The drawing under review shows one solid part. Ordinate dimensions are in mm from its lowest x, y, z. A direction names the side the tool comes from. Coordinates: 2 decimals unless noted, no trailing zeros. Order: outer loops, then holes, each group sorted by start corner. A loop starts at its lowest first (then second) coordinate and runs counter-clockwise, first axis right, second up. Notation, with made-up numbers: (-29, -12.5) - (16, -12.5) arc R31 cw to (16, 23.5) - close; hole circle Ø7 at (46.5, 84). An arc over 180 degrees is marked (long way). Answer in a Markdown table with one row per item.
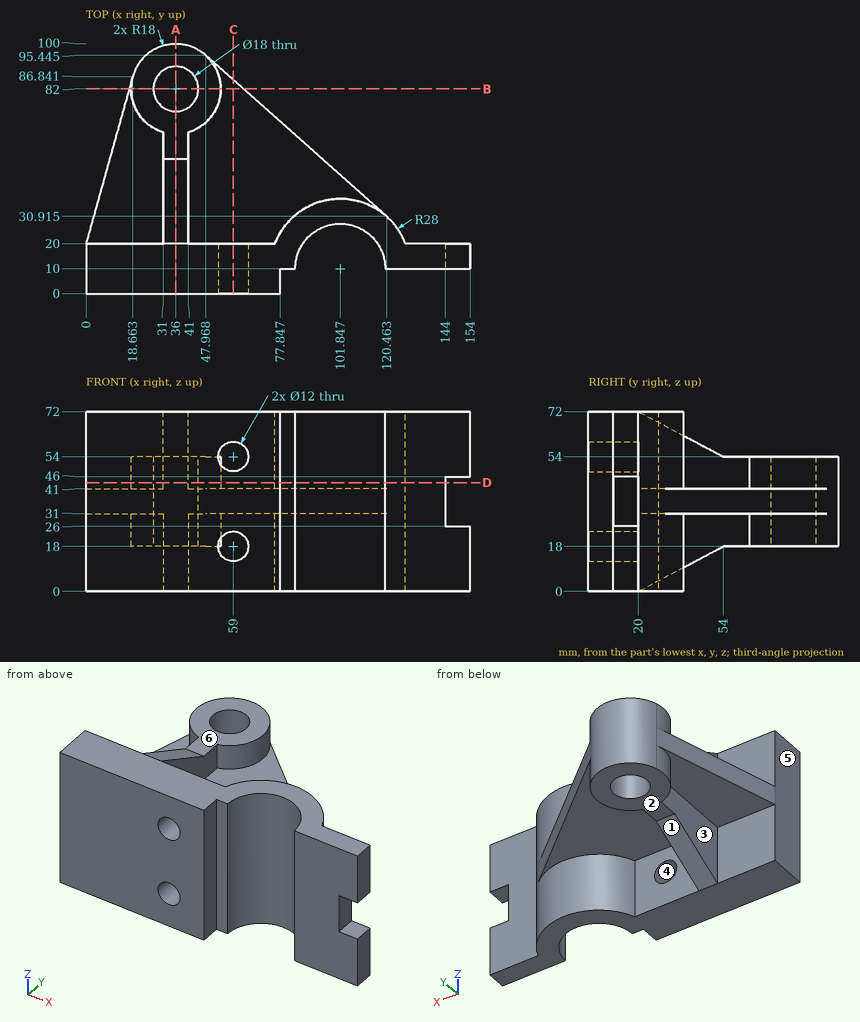
Item 1: We need section A-A, the plane x = 36. Write out the cut boundary in (y, z), then the cut area to 3 significant figures.
Check values:
| item | result |
|---|---|
| outline | (0, 0) - (20, 0) - (54, 18) - (73, 18) - (73, 54) - (54, 54) - (20, 72) - (0, 72) - close; (91, 18) - (100, 18) - (100, 54) - (91, 54) - close |
| area | 4,280 mm^2 |
Item 2: To check wall thickness, follow line 1 (Z direction, x = 59, y = 10); line 2 (Z direction, x = 55.5, y = 19.5) (1 decimal); line 3 (Y direction, x = 36, z = 41). State the ranges of each line that lie inside material, in increasing order. Write a range as from..to.
Check values:
| item | result |
|---|---|
| line 1 | 0..12, 24..48, 60..72 |
| line 2 | 0..13.1, 22.9..49.1, 58.9..72 |
| line 3 | 0..73, 91..100 |
Item 3: Tool access review of the marked faces 1, 2 and 3: name each direction out of +Z, -Z, +X, -X, +Y, -Y from which nothing blocks a thin tool from reaching the whole face with its end or side.
Check values:
| item | result |
|---|---|
| face 1 | -Z, -X, +Y |
| face 2 | -Z, +X, -X, +Y |
| face 3 | -Z, -X |
Item 4: We need section D-D, the plane z = 43.5. Write out the cut boundary in (x, y) (1 decimal), then the cut area to 3 significant figures.
Check values:
| item | result |
|---|---|
| outline | (0, 0) - (77.8, 0) - (77.8, 10) - (83.8, 10) arc R18 cw to (119.8, 10) - (144, 10) - (144, 20) - (128, 20) arc R28 ccw to (75.7, 20) - (41, 20) - (41, 64.7) arc R18 ccw (long way) to (31, 64.7) - (31, 20) - (0, 20) - close; hole circle Ø18 at (36, 82) |
| area | 3,600 mm^2 |
Item 5: We need section C-C, the plane x = 59. Write out the cut boundary in (y, z) (1 decimal), then the cut area to 3 significant figures.
Check values:
| item | result |
|---|---|
| outline | (0, 0) - (20, 0) - (20, 12) - (0, 12) - close; (0, 24) - (20, 24) - (20, 31) - (85.6, 31) - (85.6, 41) - (20, 41) - (20, 48) - (0, 48) - close; (0, 60) - (20, 60) - (20, 72) - (0, 72) - close |
| area | 1,620 mm^2 |
Item 6: We need section B-B, the plane y = 82. Write out the cut boundary in (x, z).
Check values:
| item | result |
|---|---|
| outline | (17.31, 31) - (18, 31) - (18, 18) - (27, 18) - (27, 54) - (18, 54) - (18, 41) - (17.31, 41) - close; (45, 18) - (54, 18) - (54, 31) - (63.07, 31) - (63.07, 41) - (54, 41) - (54, 54) - (45, 54) - close |
Item 7: Clearance check with flat-ended pins moving along their axes: pin 1 Ø25 at (y, z) = (50.5, 50) entering from -X (1 decimal); pin 2 Ø15.5 at (y, z) = (40, 8.5) entering from +X (1 decimal); pin 3 Ø3 at (x, z) = (134, 63.5) entering from -Y. State where each tip first meets the part, or that it passes through.
Check values:
| item | result |
|---|---|
| pin 1 | x = 6.1 |
| pin 2 | x = 118.8 |
| pin 3 | y = 10 |
Item 8: Mouldability with a two-part tool opening along X and no side actions: class the marked faces 4, 5 and 6 as +X half, -X half, draft (parallel to the pull), parting line (faces both ways), or undercut.
Check values:
| item | result |
|---|---|
| face 4 | undercut |
| face 5 | -X half |
| face 6 | draft |
